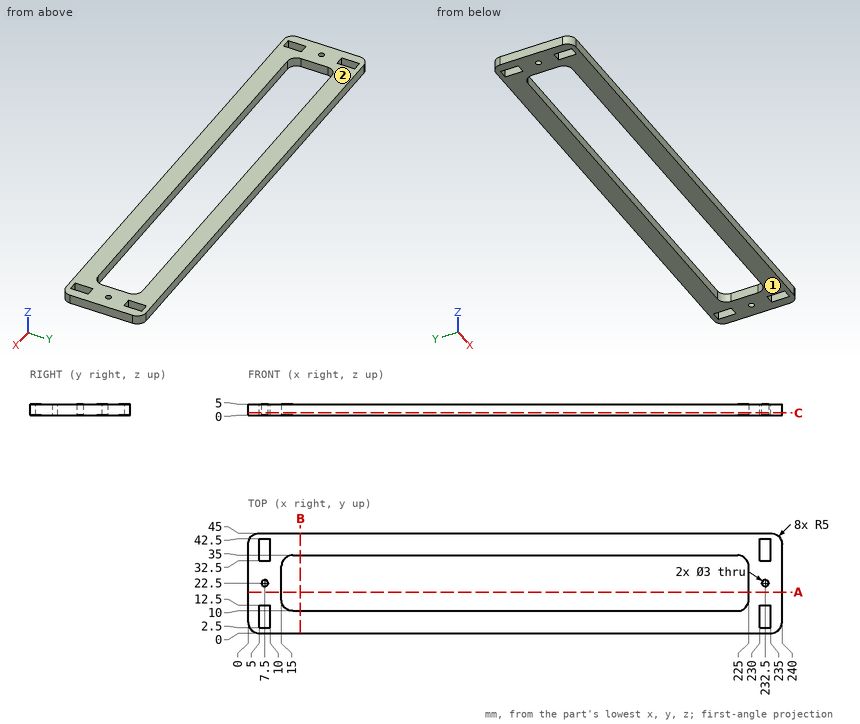
Job drawing, mm, ordinate dimensions from the low corner. One solid piece. Coordinates: 2 decimals unless noted, no trailing zeros. Write each loop counter-clockwise with the first axis right and the second up, starting at its lowest first coordinate (ties: lowest second). Pieces come first, ordered by that corner, then holes.
Item 1: Slice it at B-B (x = 23.5). Write the cut outline in (y, z), and give its area (3 significant figures).
Item 2: Slice it at A-A (y = 18.5). Write the cut outline in (x, z), and give its area (3 significant figures).
Item 3: Slice it at C-C (z = 1). Count the separate pieces of the cut face and the enclosed holes in it, and give its area (3 significant figures).
Item 4: Probe line 1 (Y direction, x = 232.5, z = 3.45); line 2 (X direction, y = 7.5, z = 3.4); line 3 (X direction, y = 19.5, z = 3.1). List the from-to ranges inside material, lowest first.
Item 5: Mould opens along Z. For the marked faces 1 and 2 say: released by +Z, released by -Z, zero draft, split by the parting line, or undercut.
Results found:
1. outline: (0, 0) - (10, 0) - (10, 5) - (0, 5) - close; (35, 0) - (45, 0) - (45, 5) - (35, 5) - close
1. area: 100 mm2
2. outline: (0, 0) - (15, 0) - (15, 5) - (0, 5) - close; (225, 0) - (240, 0) - (240, 5) - (225, 5) - close
2. area: 150 mm2
3. separate pieces: 1
3. enclosed holes: 7
3. area: 5,340 mm2
4. line 1: y = 0 to 2.5, 12.5 to 21, 24 to 32.5, 42.5 to 45
4. line 2: x = 0 to 5, 10 to 230, 235 to 240
4. line 3: x = 0 to 15, 225 to 240
5. face 1: released by -Z
5. face 2: released by +Z
